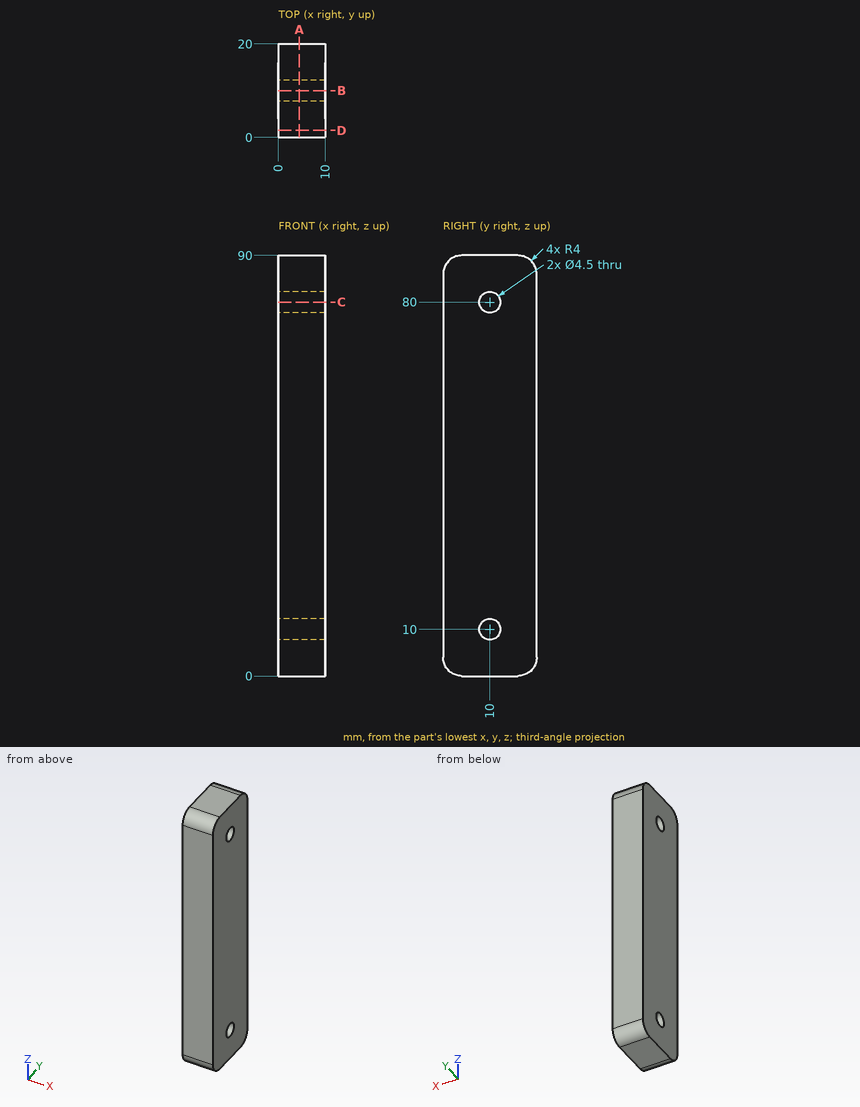
Study the drawing (mm; zero at the part's minimum x, y, z) and answer. Coordinates: 2 decimals unless noted, no trailing zeros. Order: outer loops, then holes, each group sorted by start corner. A loop starts at its lowest first (then second) coordinate and runs counter-clockwise, first axis right, second up. Notation, with made-up numbers: M 3.5,-16.5 L 22.5,-16.5 A24 ccw 22.5,15.5 Z; hole C 52,-9 d3. An arc over 180 degrees is marked long. Answer as a JSON object with one key per item and string values. Group by question number.
1. Section D-D on y = 1.5 is taken. Write down the section's boundary in (x, z).
2. Straight lines are drawn through the part: line 1 (Z direction, x = 2.5, y = 10); line 2 (Y direction, x = 4, z = 80); line 3 (Y direction, x = 7.25, z = 81). For each, find the intervals that lie inside material, in ascending order.
3. Section A-A on x = 4.5 is taken. Write down the section's boundary in (y, z), then the cut area to 3 significant figures.
4. A flat-ended cylindrical pin translates along its axis: P1, Ø3.5, axis at y = 10, z = 10, coming from the +X side. Find the tip coordinate at first contact, or state that the pin passes through.
5. Section B-B on y = 10 is taken. Write down the section's boundary in (x, z).
6. Section C-C on z = 80 is taken. Write down the section's boundary in (x, y), then the cut area to 3 significant figures.
Values follow:
{
 "1": {"outline": "M 0,0.88 L 10,0.88 L 10,89.12 L 0,89.12 Z"},
 "2": {"line 1": "0 to 7.75, 12.25 to 77.75, 82.25 to 90", "line 2": "0 to 7.75, 12.25 to 20", "line 3": "0 to 7.98, 12.02 to 20"},
 "3": {"outline": "M 0,4 A4 ccw 4,0 L 16,0 A4 ccw 20,4 L 20,86 A4 ccw 16,90 L 4,90 A4 ccw 0,86 Z; hole C 10,10 d4.5; hole C 10,80 d4.5", "area": "1,750 mm2"},
 "4": {"P1": "through"},
 "5": {"outline": "M 0,0 L 10,0 L 10,7.75 L 0,7.75 Z; M 0,12.25 L 10,12.25 L 10,77.75 L 0,77.75 Z; M 0,82.25 L 10,82.25 L 10,90 L 0,90 Z"},
 "6": {"outline": "M 0,0 L 10,0 L 10,7.75 L 0,7.75 Z; M 0,12.25 L 10,12.25 L 10,20 L 0,20 Z", "area": "155 mm2"}
}
